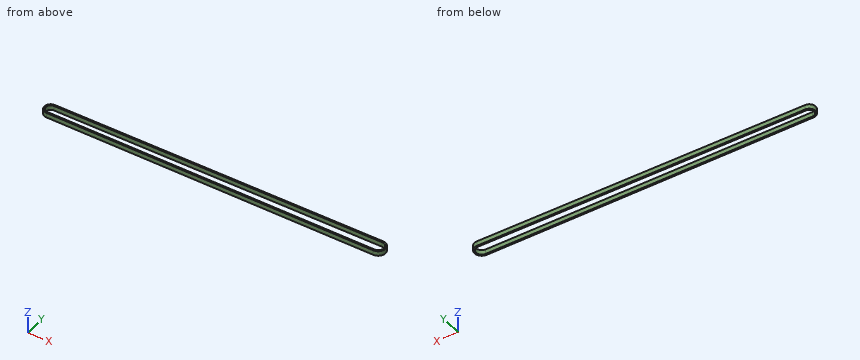
Solid Edge part; units mm, degrees
sketch "Sketch1" plane through (0, 0, 0) normal (0, 0, 1) x (1, 0, 0)
  line L0 (-32.5171, 23.9) -> (383.7412, 22.7001)
  line L1 (383.7412, 37.2999) -> (-32.5171, 36.1)
  arc A0 (383.7412, 37.2999) -> (383.7412, 22.7001) centre (383.7833, 30) cw
  arc A1 (-32.5171, 23.9) -> (-32.5171, 36.1) centre (-32.5198, 30) cw
  line L2 (-32.5198, 21.9) -> (383.7327, 20.7001)
  arc A2 (383.7327, 20.7001) -> (383.7327, 39.2999) centre (383.7833, 30) ccw
  line L3 (383.7327, 39.2999) -> (-32.5198, 38.1)
  arc A3 (-32.5198, 38.1) -> (-32.5198, 21.9) centre (-32.5198, 30) ccw
extrude "Protrusion1" add sketch "Sketch1" against normal blind 6
properties material "Polyurethene"
Can you work these out from the model? Positions are in its coordinate system, mm. Give positions to 0.01 mm unless a question says otherwise; leave off trailing zeros. Loops run counter-clockwise (first coordinate to the right, second up) from the corner with the lowest first, then second, coordinate; pieces in that order, holes last. Notation, with made-up numbers: (62.5, -20.75) - (104.5, -20.75) arc R29 cw to (104.5, 11.25) - close; hole circle Ø8 at (73, 59.25). An arc over 180 degrees is marked (long way). Return JSON: item names as keys, results as strings.
1. I'm going to push flat-ended pins straight in: pin 1 Ø3 at (y, z) = (26, -3.5) entering from -X; pin 2 Ø1 at (x, z) = (67.5, -2) entering from +Y; pin 3 Ø1 at (x, z) = (209.5, -1) entering from -Y; pin 4 Ø2 at (x, y) = (33, 36.5) entering from +Z. Where does each tip first touch, or does it pass through?
Output values:
{"pin 1": "stops at x = -40.22", "pin 2": "stops at y = 38.39", "pin 3": "stops at y = 21.2", "pin 4": "stops at z = 0"}
2. If I drill on line 1 (X direction, y = 30.5, z = -1.75); line 2 (X direction, y = 34, z = -2.1); line 3 (Y direction, x = 72, z = -4.05), over which ranges is the centre line in solid material (lowest first)?
Output values:
{"line 1": "x = -40.6 to -38.6, 391.07 to 393.07", "line 2": "x = -39.56 to -37.13, 389.89 to 392.18", "line 3": "y = 21.6 to 23.6, 36.4 to 38.4"}
3. I want a section at B-B on y = 30. Please give me the cut outline in (x, z).
Output values:
{"outline": "(-40.62, -6) - (-38.62, -6) - (-38.62, 0) - (-40.62, 0) - close; (391.08, -6) - (393.08, -6) - (393.08, 0) - (391.08, 0) - close"}
4. I want a section at C-C on x = 286. Please give me the cut outline in (y, z).
Output values:
{"outline": "(20.98, -6) - (22.98, -6) - (22.98, 0) - (20.98, 0) - close; (37.02, -6) - (39.02, -6) - (39.02, 0) - (37.02, 0) - close"}
5. I want a section at A-A on z = -2.4. Please give me the cut outline in (x, y).
Output values:
{"outline": "(-32.52, 21.9) - (383.73, 20.7) arc R9.3 ccw (long way) to (383.73, 39.3) - (-32.52, 38.1) arc R8.1 ccw to start; hole (-32.52, 23.9) - (383.74, 22.7) arc R7.3 ccw (long way) to (383.74, 37.3) - (-32.52, 36.1) arc R6.1 ccw to start"}
